from build123d import *

# Parameters (mm, degrees)
SKETCH1_R           = 520
BOSS_EXTRUDE2_DEPTH = 20
CUT_EXTRUDE2_START  = -80
SKETCH5_R           = 15.875
SKETCH5_R_2         = 2.007091202
SKETCH5_R_3         = 2
CUT_EXTRUDE2_DEPTH  = 151
CIRPATTERN6_COUNT   = 6


with BuildPart() as part:
    # Sketch1 → Boss-Extrude2 (new body)
    with BuildSketch(Plane(origin=(0, 0, 0), x_dir=(1, 0, 0), z_dir=(0, 1, 0))):
        with Locations(Location((0, 0, 0), (0, 0, 270))):
            Circle(SKETCH1_R)
    extrude(amount=BOSS_EXTRUDE2_DEPTH)

    # Sketch5 → Cut-Extrude2 (cut)
    with BuildSketch(Plane(origin=(0, 20, 0), x_dir=(1, 0, 0), z_dir=(0, 1, 0)).offset(CUT_EXTRUDE2_START)):
        with Locations(Location((0, 0, 0), (0, 0, 270))):
            Circle(SKETCH5_R)
        with Locations(Location((-439.5310312, -160.737278228, 0), (0, 0, 270))):
            Circle(SKETCH5_R_2)
        with Locations(Location((-453.620726539, -165.883197509, 0), (0, 0, 270))):
            Circle(SKETCH5_R_3)
    cut_extrude2 = extrude(amount=CUT_EXTRUDE2_DEPTH, mode=Mode.SUBTRACT)

    # CirPattern6: Cut-Extrude2 ×6 about axis
    cirpattern6_axis = Axis((0, 0, 0), (0, 1, 0))
    for i in range(1, CIRPATTERN6_COUNT):
        add(cut_extrude2.rotate(cirpattern6_axis, i * 360 / CIRPATTERN6_COUNT), mode=Mode.SUBTRACT)


solid = part.part
Here's how the part is built. I have some questions about the finished solid (model axes, mm). Round coordinates to 2 decimals unless told otherwise and drop trailing zeros. Write each loop counter-clockwise with the first axis right and the second up, starting at its lowest first coordinate (ties: lowest second). Pieces come first, ordered by that corner, then holes.
1. Suppose I cut it at A-A (x = 0). List the corners of the cut face in (y, z) for me (3 decimals).
2. Suppose I cut it at C-C (y = 11). State how many separate pieces and enclosed holes the cut face has, and give its area (3 significant figures).
3. I need wall thicknesses on L1, parallel to Z at x = 129, y = 11; L2, parallel to Z at x = 191, y = 10.75; L3, parallel to X at y = 9.75, z = -157. Which ranges of each line are inside material? Lowest first, please.
4. If we mould it in two halves opening along Z, with no side actions, what happens to faces 1 (the cylindrical face through (156.19, 9.86, 495.99)), 2 (the flat face through (7, 20, 108)), 3 (the cylindrical face through (-15.497, 9.86, -3.441))? For each: released by +Z, released by -Z, zero draft, split by the parting line, or undercut.
5. Will these pins go through, and if not, where does the flat tip stop? pin 1 Ø6 at (x, y) = (-102.5, 6) entering from +Z; pin 2 Ø1 at (x, y) = (413.5, 16) entering from -Z; pin 3 Ø5 at (y, z) = (4.5, 84) entering from +X.
6. Suppose I cut it at D-D (x = 104). List the corners of the cut face in (y, z) for me, and give its area (3 significant figures).
7. Suppose I cut it at B-B (z = 0). List the corners of the cut face in (x, y) for me (3 decimals), and give its area (3 significant figures).
Answer sheet:
1. outline: (0, -520) - (20, -520) - (20, -15.875) - (0, -15.875) - close; (0, 15.875) - (20, 15.875) - (20, 520) - (0, 520) - close
2. separate pieces: 1
2. enclosed holes: 13
2. area: 849,000 mm2
3. L1: z = -503.74 to 503.74
3. L2: z = -483.65 to 483.65
3. L3: x = -495.73 to 495.73
4. face 1: split by the parting line
4. face 2: zero draft
4. face 3: undercut
5. pin 1: stops at z = 510.39
5. pin 2: stops at z = -315.96
5. pin 3: stops at x = 513.57
6. outline: (0, -509.49) - (20, -509.49) - (20, 509.49) - (0, 509.49) - close
6. area: 20,400 mm2
7. outline: (-520, 0) - (-15.875, 0) - (-15.875, 20) - (-520, 20) - close; (15.875, 0) - (520, 0) - (520, 20) - (15.875, 20) - close
7. area: 20,200 mm2
